from build123d import *

# Parameters (mm, degrees)
SKETCH008_W     = 125
SKETCH008_H     = 55
PAD008_DEPTH    = 100
SKETCH010_W     = 115
SKETCH010_H     = 25
POCKET_DEPTH    = 60
SKETCH011_W     = 115
SKETCH011_H     = 20
POCKET001_DEPTH = 50
SKETCH012_W     = 115
SKETCH012_H     = 46
POCKET002_DEPTH = 53


with BuildPart() as part:
    # Sketch008 → Pad008 (new body)
    with BuildSketch(Plane.XY):
        Rectangle(SKETCH008_W, SKETCH008_H)
    extrude(amount=PAD008_DEPTH)

    # Sketch010 → Pocket (cut)
    with BuildSketch(Plane(origin=(0, 27.5, 0), x_dir=(-1, 0, 0), z_dir=(0, 1, 0))):
        with Locations((0, 12.5)):
            Rectangle(SKETCH010_W, SKETCH010_H)
    extrude(amount=-POCKET_DEPTH, mode=Mode.SUBTRACT)

    # Sketch011 → Pocket001 (cut)
    with BuildSketch(Plane(origin=(0, 27.5, 0), x_dir=(-1, 0, 0), z_dir=(0, 1, 0))):
        with Locations((0, 35)):
            Rectangle(SKETCH011_W, SKETCH011_H)
    extrude(amount=-POCKET001_DEPTH, mode=Mode.SUBTRACT)

    # Sketch012 → Pocket002 (cut)
    with BuildSketch(Plane(origin=(0, 0, 45), x_dir=(1, 0, 0), z_dir=(0, 0, -1))):
        Rectangle(SKETCH012_W, SKETCH012_H)
    extrude(amount=-POCKET002_DEPTH, mode=Mode.SUBTRACT)


solid = part.part
Geometry check sheet. Reference: the model listing, model coordinates, mm. A direction names the side the tool comes from. Give positions to 0.01 mm unless a question says otherwise; leave off trailing zeros. Write each loop counter-clockwise with the first axis right and the second up, starting at its lowest first coordinate (ties: lowest second). Pieces come first, ordered by that corner, then holes. Notation, with made-up numbers: (85, 10.25) - (112, 10.25) arc R29 ccw to (112, 41.25) - close; hole circle Ø8 at (52, 42). An arc over 180 degrees is marked (long way). Put each result on its own line as item: value.
1. Set-up check for faces 1 (the flat face through (1, -25, 25)), 2 (the flat face through (1, -22.5, 35)), 3 (the flat face through (-1, 27.5, 72)), 4 (the flat face through (-60, 0, 0)), 5 (the flat face through (-1, 23, 71)): record each of +Z, -Z, +X, -X, +Y, -Y from which the full face is reachable in a straight line by a thin tool's end or side.
Ans:
face 1: -Z, +Y, -Y
face 2: -Z, +Y
face 3: +Z, -Z, +X, -X, +Y
face 4: -Z, +X, -X, +Y, -Y
face 5: -Z
2. Thickness scan on line 1 (Y direction, x = 30.5, z = 79.5); line 2 (X direction, y = 11.5, z = 56); line 3 (Y direction, x = 23.5, z = 35). Record the ranges inside material, lowest first.
Ans:
line 1: y = -27.5 to -23, 23 to 27.5
line 2: x = -62.5 to -57.5, 57.5 to 62.5
line 3: y = -27.5 to -22.5
3. Sectioned sample at A-A, the plane z = 16. Enter the section's corners in (x, y).
Ans:
outline: (-62.5, -27.5) - (-57.5, -27.5) - (-57.5, 27.5) - (-62.5, 27.5) - close; (57.5, -27.5) - (62.5, -27.5) - (62.5, 27.5) - (57.5, 27.5) - close
4. Sectioned sample at B-B, the plane x = -33.5. Enter the section's corners in (y, z), plus the area to 3 significant figures.
Ans:
outline: (-27.5, 25) - (-22.5, 25) - (-22.5, 45) - (-23, 45) - (-23, 98) - (23, 98) - (23, 45) - (27.5, 45) - (27.5, 100) - (-27.5, 100) - close
area: 687 mm²
5. Draft check along X on faces 6 (the flat face through (-1, -27.5, 60)), 7 (the flat face through (-62.5, 0, 49)), 8 (the flat face through (62.5, 0, 49)), 9 (the flat face through (-1, -23, 71)). Enter one of: +X half, -X half, draft (parallel to the pull), parting line (faces both ways), or undercut.
Ans:
face 6: draft
face 7: -X half
face 8: +X half
face 9: undercut
6. Go/stop test with flat-tipped pins: pin 1 (10 mm diameter, centred on x = 9, z = 31.5, fed in from +Y); pin 2 (8 mm diameter, centred on x = -6, y = 15, fed in from -Z); pin 3 (2 mm diameter, centred on x = 16.5, y = 25.5, fed in from -Z). Record where each tip stops, or that it passes through.
Ans:
pin 1: stops at y = -22.5
pin 2: stops at z = 98
pin 3: stops at z = 45
7. Sectioned sample at C-C, the plane y = 10.5. Enter the section's corners in (x, z), plus the area to 3 significant figures.
Ans:
outline: (-62.5, 0) - (-57.5, 0) - (-57.5, 98) - (57.5, 98) - (57.5, 0) - (62.5, 0) - (62.5, 100) - (-62.5, 100) - close
area: 1,230 mm²
8. Sectioned sample at D-D, the plane z = 51. Enter the section's corners in (x, y).
Ans:
outline: (-62.5, -27.5) - (62.5, -27.5) - (62.5, 27.5) - (-62.5, 27.5) - close; hole (-57.5, -23) - (57.5, -23) - (57.5, 23) - (-57.5, 23) - close
